Here's how the part is built. I have some questions about the finished solid (model axes, mm). A direction names the side the tool comes from. Give positions to 0.01 mm unless a question says otherwise; leave off trailing zeros. Write each loop counter-clockwise with the first axis right and the second up, starting at its lowest first coordinate (ties: lowest second). Pieces come first, ordered by that corner, then holes. Notation, with made-up numbers: (9, 29.5) -> (49, 29.5) arc R34 cw to (49, 60.5) -> close; hole circle Ø2 at (-39.75, 5.5). An arc over 180 degrees is marked (long way). Use CSV: the item, a comma, the result in double quotes. Start each with the question number.
(1) Suppose I cut it at B-B on x = 0. List the corners of the cut face in (y, z) for me, plus the area to 3 significant figures.
(2) Which directions (+Z, -Z, +X, -X, +Y, -Y) give clear straight access to the entire face, cutting with the end or side of a thin tool? Please do faces 4 (the flat face through (2, 0, 8)), 5 (the flat face through (5, -11, 7.5)), 6 (the flat face through (0, 0, 5)).
(3) I need wall thicknesses on L1, parallel to Y at x = 0, z = 1.6; L2, parallel to Y at x = 0, z = 7.7; L3, parallel to Z at x = 1.5, y = 2.5. Which ranges of each line are inside material? Lowest first, please. Write a range as [from, to].
(4) Suppose I cut it at A-A on z = 2. List the corners of the cut face in (x, y) for me, plus the area to 3 significant figures.
(5) For pin 1 Ø0.6 at (y, z) = (3, 8) entering from -X; pin 2 Ø1 at (x, z) = (-1.5, 5.5) entering from +Y; pin 3 Ø3 at (y, z) = (-5, 1.5) entering from +X, each with a flat end and sliding along its axis, tell me the tip position at first contact or that it passes through.
(6) If we mould it in two halves opening along X, with no side actions, what happens to faces 1 (the flat face through (6, 0, 0)), 2 (the cylindrical face through (-2.4, -4.5, 2.7)), 3 (the cylindrical face through (12.932, -5.362, 3.951))? For each: pulls with the +X half, pulls with the -X half, needs draft (parallel to the pull), parting line crosses it, or undercut.
(7) Suppose I cut it at C-C on z = 7. List the corners of the cut face in (x, y) for me, plus the area to 3 significant figures.
from build123d import *

# Parameters (mm, degrees)
SKETCH_1_R          = 14
EXTRUDE_1_DEPTH     = 8
SKETCH_2_R          = 13
SKETCH_2_R_2        = 11.5
CUT_EXTRUDE_1_DEPTH = 0.5
SKETCH_3_R          = 5.1
CUT_EXTRUDE_2_DEPTH = 5
CHAMFER_1_SIZE      = 0.5
FILLET_1_R          = 0.5
CUT_EXTRUDE_3_DEPTH = 0.5


with BuildPart() as part:
    # 草图1 → 凸台-拉伸1 (new body)
    with BuildSketch(Plane.XY):
        Circle(SKETCH_1_R)
    extrude(amount=EXTRUDE_1_DEPTH)

    # 草图2 → 切除-拉伸1 (cut)
    with BuildSketch(Plane.XY.offset(8)):
        Circle(SKETCH_2_R)
        Circle(SKETCH_2_R_2, mode=Mode.SUBTRACT)
    extrude(amount=-CUT_EXTRUDE_1_DEPTH, mode=Mode.SUBTRACT)

    # 草图3 → 切除-拉伸2 (cut)
    with BuildSketch(Plane(origin=(0, 0, 0), x_dir=(-1, 0, 0), z_dir=(0, 0, -1))):
        Circle(SKETCH_3_R)
    extrude(amount=-CUT_EXTRUDE_2_DEPTH, mode=Mode.SUBTRACT)

    # 倒角1
    chamfer_1_edges = [part.edges().sort_by_distance(p)[0] for p in [
        (5.1, 0, 0),
    ]]
    chamfer(chamfer_1_edges, length=CHAMFER_1_SIZE)

    # 圆角1
    fillet_1_edges = [part.edges().sort_by_distance(p)[0] for p in [
        (-14, 0, 0),
        (-14, 0, 8),
    ]]
    fillet(fillet_1_edges, radius=FILLET_1_R)

    # 草图4 → 切除-拉伸3 (cut)
    with BuildSketch(Plane.XY.offset(8)):
        with BuildLine():
            Line((-0.332439592, 1.750042466), (-0.360140423, 5.733421968))
            add(Edge.make_bspline(
                [(-0.360140423, 5.733421968), (-0.361352645, 5.905161235), (-0.363614161, 6.225557253), (-0.362563714, 6.6716641), (-0.376473853, 7.047374008), (-0.385330649, 7.359666935), (-0.402429288, 7.62108814), (-0.424047197, 7.845666351), (-0.450655997, 8.039057288), (-0.486147264, 8.214138322), (-0.538863863, 8.394313463), (-0.604319105, 8.608623265), (-0.69811297, 8.866152605), (-0.768099985, 9.052974569), (-0.806123802, 9.154474599)],
                knots=[0, 0, 0, 0, 1.776080644, 3.313448207, 4.612630616, 5.663679929, 6.544024972, 7.321231433, 7.996425259, 8.561978184, 9.16664432, 9.936779763, 10.879056232, 12, 12, 12, 12], degree=3))
            Line((-0.806123802, 9.154474599), (-0.529115492, 9.398241912))
            Line((-0.529115492, 9.398241912), (1.28528894, 7.977189281))
            add(Edge.make_bspline(
                [(1.28528894, 7.977189281), (1.212689416, 7.888764213), (1.076355109, 7.72271119), (0.907905181, 7.473619686), (0.778857884, 7.248302871), (0.690090199, 7.028698577), (0.643415827, 6.786186198), (0.597023873, 6.498405776), (0.567426595, 6.145605356), (0.545007238, 5.747427005), (0.525356606, 5.343894899), (0.516092277, 4.972576481), (0.505970295, 4.653140232), (0.504704552, 4.457343357), (0.504125505, 4.367770998)],
                knots=[0, 0, 0, 0, 1.084774512, 2.037092997, 2.848708899, 3.544871268, 4.271658147, 5.184656451, 6.310726112, 7.626940673, 8.968471314, 10.142701689, 11.150330718, 12, 12, 12, 12], degree=3))
            Line((0.504125505, 4.367770998), (0.504125505, 1.82483471))
            Line((0.504125505, 1.82483471), (3.321300021, 2.124003685))
            add(Edge.make_bspline(
                [(3.321300021, 2.124003685), (3.42652928, 2.139025527), (3.663624238, 2.172871655), (4.057608853, 2.222727844), (4.527947814, 2.292502711), (5.058622387, 2.362973897), (5.614072784, 2.456659085), (6.154444434, 2.587180098), (6.664734902, 2.745631608), (6.986142322, 2.880481389), (7.144014702, 2.946718367)],
                knots=[0, 0, 0, 0, 0.649902526, 1.464313377, 2.427986904, 3.556930783, 4.73754275, 5.869953849, 6.953740843, 8, 8, 8, 8], degree=3))
            Line((7.144014702, 2.946718367), (8.035981461, 2.254197591))
            add(Edge.make_bspline(
                [(8.035981461, 2.254197591), (8.080959366, 2.220886663), (8.159539314, 2.162689843), (8.252827302, 2.077830082), (8.307983989, 2.009717031), (8.321391828, 1.94420007), (8.283079852, 1.900605024), (8.222569166, 1.879078168), (8.138400359, 1.862528273), (8.073037414, 1.861454526), (8.035981461, 1.86084579)],
                knots=[0, 0, 0, 0, 1.835156804, 3.206163717, 4.12161621, 4.700123913, 5.196760664, 5.860863374, 6.787267836, 8, 8, 8, 8], degree=3))
            Line((8.035981461, 1.86084579), (7.227117195, 1.844225292))
            Line((7.227117195, 1.844225292), (6.362851267, 1.750042466))
            Line((6.362851267, 1.750042466), (0.504125505, 1.112923353))
            Line((0.504125505, 1.112923353), (0.504125505, -5.878766398))
            Line((0.504125505, -5.878766398), (1.368391433, -5.803974154))
            add(Edge.make_bspline(
                [(1.368391433, -5.803974154), (1.561462147, -5.786385303), (1.935094465, -5.752347189), (2.474534057, -5.688787282), (2.974290009, -5.617039302), (3.434533274, -5.537557716), (3.854668132, -5.448672356), (4.23555044, -5.356628694), (4.575244967, -5.252223674), (4.784345257, -5.169921401), (4.88362689, -5.13084396)],
                knots=[0, 0, 0, 0, 1.29553906, 2.507139754, 3.629368228, 4.669195067, 5.627680362, 6.498691998, 7.287173099, 8, 8, 8, 8], degree=3))
            Line((4.88362689, -5.13084396), (5.775593649, -5.803974154))
            add(Edge.make_bspline(
                [(5.775593649, -5.803974154), (5.817072398, -5.83713927), (5.888656192, -5.894375444), (5.971238583, -5.979775819), (6.02161762, -6.04253168), (6.035824152, -6.104047047), (5.996806703, -6.143717178), (5.936119537, -6.162435734), (5.850855599, -6.175102485), (5.784876091, -6.176917826), (5.747892818, -6.177935373)],
                knots=[0, 0, 0, 0, 1.812194932, 3.127475989, 4.036720824, 4.576297278, 5.068692798, 5.747705924, 6.737529143, 8, 8, 8, 8], degree=3))
            Line((5.747892818, -6.177935373), (5.301909439, -6.197325955))
            Line((5.301909439, -6.197325955), (4.520746004, -6.233337035))
            Line((4.520746004, -6.233337035), (3.628779245, -6.327519861))
            Line((3.628779245, -6.327519861), (2.121854037, -6.457713766))
            Line((2.121854037, -6.457713766), (-1.141303857, -6.740262243))
            add(Edge.make_bspline(
                [(-1.141303857, -6.740262243), (-1.255758527, -6.754469707), (-1.47626363, -6.781841404), (-1.794394083, -6.815523946), (-2.0867365, -6.853615725), (-2.354021003, -6.884446926), (-2.596232118, -6.920650211), (-2.813843434, -6.945556544), (-3.005595903, -6.974642338), (-3.23226146, -7.007828608), (-3.510911328, -7.055457968), (-3.858422546, -7.129968972), (-4.235310728, -7.213583069), (-4.494280475, -7.283092979), (-4.628838483, -7.319209611)],
                knots=[0, 0, 0, 0, 1.173024538, 2.259915622, 3.253542956, 4.171454364, 4.996242764, 5.744084598, 6.39886201, 6.968650651, 8.074127918, 9.273179876, 10.583172403, 12, 12, 12, 12], degree=3))
            Line((-4.628838483, -7.319209611), (-5.410001918, -6.740262243))
            add(Edge.make_bspline(
                [(-5.410001918, -6.740262243), (-5.450722452, -6.709069955), (-5.521636813, -6.654748927), (-5.61115149, -6.583007343), (-5.666823555, -6.533702581), (-5.697711988, -6.484415815), (-5.674943077, -6.430258701), (-5.649144053, -6.4001522), (-5.63437865, -6.382921523)],
                knots=[0, 0, 0, 0, 1.845274552, 3.213525351, 4.10520704, 4.550429949, 5.170376093, 6, 6, 6, 6], degree=3))
            Line((-5.63437865, -6.382921523), (-4.293658428, -6.327519861))
            Line((-4.293658428, -6.327519861), (-2.983409121, -6.216716536))
            Line((-2.983409121, -6.216716536), (-0.360140423, -5.953558642))
            Line((-0.360140423, -5.953558642), (-0.360140423, 1.038131109))
            Line((-0.360140423, 1.038131109), (-1.700860644, 0.871926123))
            Line((-1.700860644, 0.871926123), (-2.426622417, 0.777743297))
            add(Edge.make_bspline(
                [(-2.426622417, 0.777743297), (-2.701812878, 0.737311731), (-3.227393674, 0.660092285), (-3.978116975, 0.546657661), (-4.653090311, 0.441375307), (-5.252805162, 0.34603544), (-5.775671732, 0.252487806), (-6.224429528, 0.175191604), (-6.596059424, 0.099410354), (-6.818167512, 0.051239755), (-6.916927126, 0.02982086)],
                knots=[0, 0, 0, 0, 1.466159973, 2.800189808, 4.002110139, 5.067144397, 6.000968071, 6.801993663, 7.467310513, 8, 8, 8, 8], degree=3))
            Line((-6.916927126, 0.02982086), (-7.781193054, 0.702951054))
            add(Edge.make_bspline(
                [(-7.781193054, 0.702951054), (-7.813806148, 0.724644837), (-7.87162741, 0.763106747), (-7.941670689, 0.817660634), (-7.986665168, 0.854457065), (-8.012472353, 0.892884107), (-7.995931201, 0.936594338), (-7.984222445, 0.966501178), (-7.977868954, 0.982729447)],
                knots=[0, 0, 0, 0, 1.797637159, 3.187114011, 4.056246988, 4.492359064, 5.181912803, 6, 6, 6, 6], degree=3))
            Line((-7.977868954, 0.982729447), (-6.664849564, 1.076912272))
            Line((-6.664849564, 1.076912272), (-5.46540358, 1.171095098))
            Line((-5.46540358, 1.171095098), (-3.094212445, 1.431482909))
            Line((-3.094212445, 1.431482909), (-0.332439592, 1.750042466))
        make_face()
    extrude(amount=-CUT_EXTRUDE_3_DEPTH, mode=Mode.SUBTRACT)


solid = part.part
Geometry says:
1,outline,"(-14, 0.5) arc R0.5 ccw to (-13.5, 0) -> (-5.6, 0) -> (-5.1, 0.5) -> (-5.1, 5) -> (5.1, 5) -> (5.1, 0.5) -> (5.6, 0) -> (13.5, 0) arc R0.5 ccw to (14, 0.5) -> (14, 7.5) arc R0.5 ccw to (13.5, 8) -> (13, 8) -> (13, 7.5) -> (11.5, 7.5) -> (11.5, 8) -> (8.98, 8) -> (8.98, 7.5) -> (-6.64, 7.5) -> (-6.64, 8) -> (-11.5, 8) -> (-11.5, 7.5) -> (-13, 7.5) -> (-13, 8) -> (-13.5, 8) arc R0.5 ccw to (-14, 7.5) -> close"
1,area,"163 mm²"
2,face 4,"+Z, +X, -X, +Y, -Y"
2,face 5,"+Z"
2,face 6,"-Z"
3,L1,"[-14, -5.1], [5.1, 14]"
3,L2,"[-13.96, -13], [-11.5, -6.64], [8.98, 11.5], [13, 13.96]"
3,L3,"[5, 8]"
4,outline,"circle Ø28 at (0, 0); hole circle Ø10.2 at (0, 0)"
4,area,"534 mm²"
5,pin 1,"x = -13.65"
5,pin 2,"y = 13.96"
5,pin 3,"x = 13.56"
6,face 1,"needs draft"
6,face 2,"undercut"
6,face 3,"parting line crosses it"
7,outline,"circle Ø28 at (0, 0)"
7,area,"616 mm²"
